from build123d import *

# Parameters (mm, degrees)
SKETCH1_R           = 45
BOSS_EXTRUDE1_DEPTH = 20
SKETCH2_R           = 15
CUT_EXTRUDE1_DEPTH  = 21
SKETCH3_R           = 5
BOSS_EXTRUDE2_DEPTH = 220
SKETCH4_R           = 45
BOSS_EXTRUDE3_DEPTH = 20
CHAMFER1_SIZE       = 2


with BuildPart() as part:
    # Sketch1 → Boss-Extrude1 (new body)
    with BuildSketch(Plane(origin=(0, 0, 0), x_dir=(1, 0, 0), z_dir=(0, 1, 0))):
        Circle(SKETCH1_R)
    extrude(amount=BOSS_EXTRUDE1_DEPTH)

    # Sketch2 → Cut-Extrude1 (cut, through all)
    with BuildSketch(Plane(origin=(0, 20, 0), x_dir=(1, 0, 0), z_dir=(0, 1, 0))):
        Circle(SKETCH2_R)
    extrude(amount=-CUT_EXTRUDE1_DEPTH, mode=Mode.SUBTRACT)

    # Sketch3 → Boss-Extrude2 (add)
    with BuildSketch(Plane(origin=(0, 20, 0), x_dir=(1, 0, 0), z_dir=(0, 1, 0))):
        with Locations((35, 0)):
            Circle(SKETCH3_R)
        with Locations((0, -35)):
            Circle(SKETCH3_R)
        with Locations((-35, 0)):
            Circle(SKETCH3_R)
        with Locations((0, 35)):
            Circle(SKETCH3_R)
        with Locations((24.748737342, 24.748737342)):
            Circle(SKETCH3_R)
    extrude(amount=BOSS_EXTRUDE2_DEPTH)

    # Sketch4 → Boss-Extrude3 (add)
    with BuildSketch(Plane(origin=(0, 240, 0), x_dir=(1, 0, 0), z_dir=(0, 1, 0))):
        Circle(SKETCH4_R)
    extrude(amount=BOSS_EXTRUDE3_DEPTH)

    # Chamfer1
    chamfer1_edges = [part.edges().sort_by_distance(p)[0] for p in [
        (-45, 0, 0),
        (-45, 240, 0),
        (-45, 260, 0),
        (-45, 20, 0),
    ]]
    chamfer(chamfer1_edges, length=CHAMFER1_SIZE)


solid = part.part
Part model, mm, in its own coordinate system. A direction names the side the tool comes from. Give positions to 0.01 mm unless a question says otherwise; leave off trailing zeros. Loops run counter-clockwise (first coordinate to the right, second up) from the corner with the lowest first, then second, coordinate; pieces in that order, holes last.
(1) Pull direction Z, two halves, no side cores. Call faces 1 (the cylindrical face through (-1.08, 128.46, 39.88)), 2 (the cylindrical face through (20.765, 249.888, 39.923)), 3 (the flat face through (-1, 260, -1)): pulls with the +Z half, pulls with the -Z half, needs draft (parallel to the pull), parting line crosses it, or undercut.
Return value:
face 1: undercut
face 2: parting line crosses it
face 3: needs draft
(2) 3-axis set-ups, long thin cutter, end or side, ignore diameter. For faces 4 (the cylindrical face through (30, 128, 0)), 5 (the cylindrical face through (-14.985, 10.14, -0.66)), 6 (the flat face through (19, 0, -1)): which of +Z, -Z, +X, -X, +Y, -Y reach the whole face in a straight line?
Return value:
face 4: none
face 5: -Y
face 6: +Z, -Z, +X, -X, -Y
(3) Band-saw the part on C-C (y = 159). Write the cut outline in (x, z).
Return value:
outline: circle Ø10 at (-35, 0); circle Ø10 at (0, -35); circle Ø10 at (0, 35); circle Ø10 at (24.75, -24.75); circle Ø10 at (35, 0)
(4) Pin check, flat tips, straight feed: pin 1 (1 mm diameter, centred on x = 18, y = 145.5, fed in from +Z); pin 2 (12 mm diameter, centred on x = -27, y = 193.5, fed in from -Z); pin 3 (12 mm diameter, centred on x = -8, y = 80.5, fed in from -Z); pin 4 (10 mm diameter, centred on x = -1, y = 193.5, fed in from +Z). Stop position of each tip, or through.
Return value:
pin 1: passes through
pin 2: stops at z = -4.58
pin 3: stops at z = -39.58
pin 4: stops at z = 40
(5) Band-saw the part on B-B (x = 0). Write the cut outline in (y, z).
Return value:
outline: (0, -43) - (2, -45) - (18, -45) - (20, -43) - (20, -40) - (240, -40) - (240, -43) - (242, -45) - (258, -45) - (260, -43) - (260, 43) - (258, 45) - (242, 45) - (240, 43) - (240, 40) - (20, 40) - (20, 43) - (18, 45) - (2, 45) - (0, 43) - (0, 15) - (20, 15) - (20, 30) - (240, 30) - (240, -30) - (20, -30) - (20, -15) - (0, -15) - close
(6) Drill centre lines: line 1 along X through (y, z) = (4, 0); line 2 along Y through (x, z) = (-30, -26). Where is each one in solid material? Low to high.
Return value:
line 1: x = -45 to -15, 15 to 45
line 2: y = 0 to 20, 240 to 260
(7) Band-saw the part on A-A (z = 0). Write the cut outline in (x, y), and give its area (3 significant figures).
Return value:
outline: (-45, 2) - (-43, 0) - (-15, 0) - (-15, 20) - (-30, 20) - (-30, 240) - (30, 240) - (30, 20) - (15, 20) - (15, 0) - (43, 0) - (45, 2) - (45, 18) - (43, 20) - (40, 20) - (40, 240) - (43, 240) - (45, 242) - (45, 258) - (43, 260) - (-43, 260) - (-45, 258) - (-45, 242) - (-43, 240) - (-40, 240) - (-40, 20) - (-43, 20) - (-45, 18) - close
area: 7,380 mm2
